Could you check a few things on this drawing? It's one solid part, dimensions in mm from its lowest x, y, z. Give positions to 0.01 mm unless a question says otherwise; leave off trailing zeros. Loops run counter-clockwise (first coordinate to the right, second up) from the corner with the lowest first, then second, coordinate; pieces in that order, holes last. Notation, with made-up numbers: M 61,10 L 72,10 A16 ccw 72,37 Z; hole C 82.5,70 d7. An arc over 180 degrees is marked long. Answer as CSV lines item,"result". Start each with the question number.
Item 1: Will this pin go through, and if not, where does the flat tip stop? P1, Ø4, axis at x = 45, z = 32.5, coming from the -Y side.
Item 2: I want a section at B-B on y = 0.5. Give the number of separate pieces and of enclosed holes in the cut face, plus the area to 3 significant figures.
Item 3: I want a section at A-A on z = 8. List the corners of the cut face in (x, y) for me (1 decimal).
Item 4: If I drill on line 1 along X through (y, z) = (2.45, 3); line 2 along Z through (x, y) = (62.5, 2) (1 decimal); line 3 along X through (y, z) = (1.2, 33.5), over which ranges is the centre line in solid material (lowest first)? Write a range as from..to.
Item 5: I want a section at C-C on x = 55. List the corners of the cut face in (y, z) for me (1 decimal).
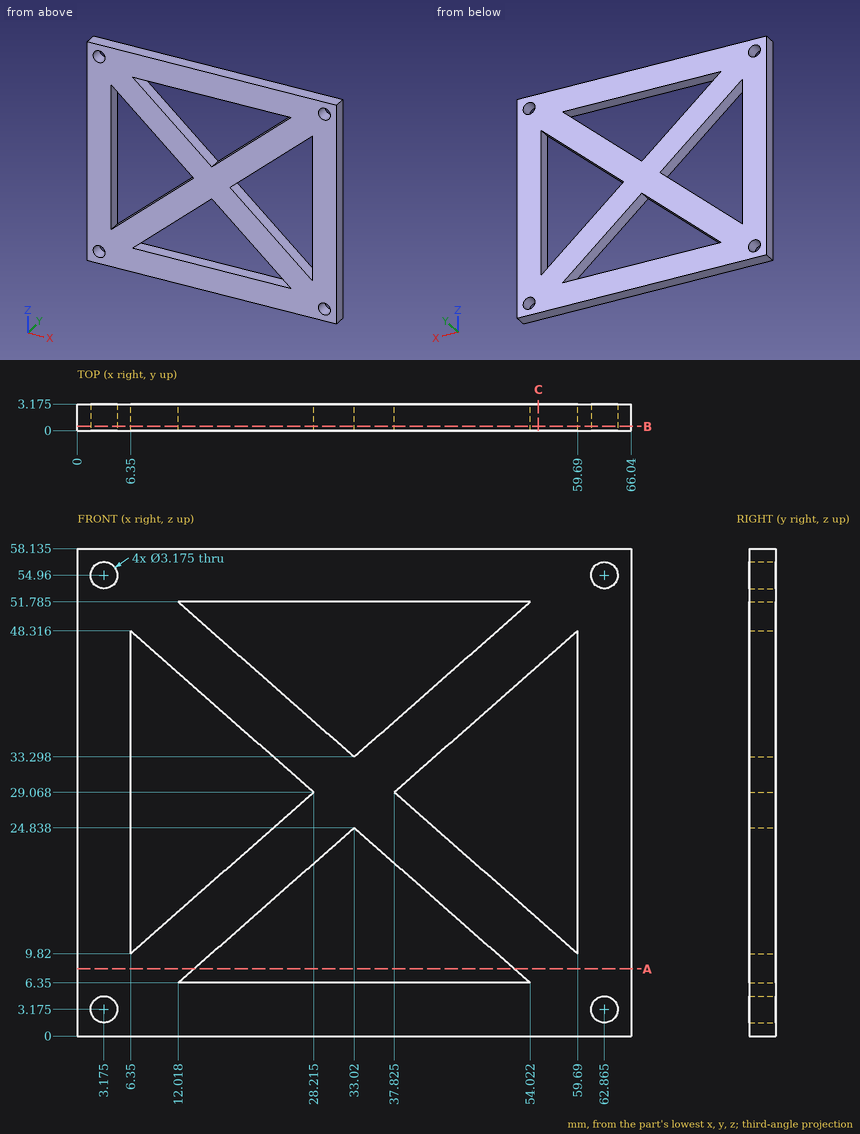
Result:
1,P1,"through"
2,separate pieces,"1"
2,enclosed holes,"8"
2,area,"2,190 mm^2"
3,outline,"M 0,0 L 13.9,0 L 13.9,3.2 L 0,3.2 Z; M 52.1,0 L 66,0 L 66,3.2 L 52.1,3.2 Z"
4,line 1,"0..1.6, 4.75..61.29, 64.44..66.04"
4,line 2,"0..1.6, 4.7..53.4, 56.5..58.1"
4,line 3,"0..6.35, 23.18..32.79, 33.25..42.86, 59.69..66.04"
5,outline,"M 0,0 L 3.2,0 L 3.2,13.9 L 0,13.9 Z; M 0,44.2 L 3.2,44.2 L 3.2,58.1 L 0,58.1 Z"
